Part model, mm, in its own coordinate system. A direction names the side the tool comes from. Give positions to 0.01 mm unless a question says otherwise; leave off trailing zeros. Order: outer loops, then holes, each group sorted by start corner. A loop starts at its lowest first (then second) coordinate and runs counter-clockwise, first axis right, second up. Notation, with made-up numbers: M -33.5,18 L -19.5,18 A25 cw -19.5,44 Z; hole C -17,-26 d2. An arc over 180 degrees is marked long. One line per question, with ' | ' between items.
```python
from build123d import *

# Parameters (mm, degrees)
SKETCH1_W           = 110
SKETCH1_H           = 45
BOSS_EXTRUDE1_DEPTH = 2
SKETCH3_W           = 110
SKETCH3_H           = 45
SKETCH3_W_2         = 106
SKETCH3_H_2         = 41
BOSS_EXTRUDE2_DEPTH = 30
SKETCH4_W           = 12
SKETCH4_H           = 41
BOSS_EXTRUDE3_DEPTH = 12
SKETCH5_W           = 6
SKETCH5_H           = 6
BOSS_EXTRUDE4_DEPTH = 18
SKETCH6_W           = 6
SKETCH6_H           = 6
BOSS_EXTRUDE5_DEPTH = 18
FILLET1_R           = 4
FILLET2_R           = 4
SKETCH7_R           = 1.3
CUT_EXTRUDE1_DEPTH  = 34
SKETCH8_R           = 2.9
CUT_EXTRUDE2_DEPTH  = 25
SKETCH9_W           = 10
SKETCH9_H           = 20
CUT_EXTRUDE3_DEPTH  = 10


with BuildPart() as part:
    # Sketch1 → Boss-Extrude1 (new body)
    with BuildSketch(Plane(origin=(0, 0, 0), x_dir=(1, 0, 0), z_dir=(0, 1, 0))):
        Rectangle(SKETCH1_W, SKETCH1_H)
    extrude(amount=BOSS_EXTRUDE1_DEPTH)

    # Sketch3 → Boss-Extrude2 (add)
    with BuildSketch(Plane(origin=(0, 2, 0), x_dir=(1, 0, 0), z_dir=(0, 1, 0))):
        Rectangle(SKETCH3_W, SKETCH3_H)
        Rectangle(SKETCH3_W_2, SKETCH3_H_2, mode=Mode.SUBTRACT)
    extrude(amount=BOSS_EXTRUDE2_DEPTH)

    # Sketch4 → Boss-Extrude3 (add)
    with BuildSketch(Plane(origin=(0, 2, 0), x_dir=(1, 0, 0), z_dir=(0, 1, 0))):
        with Locations((-47, 0)):
            Rectangle(SKETCH4_W, SKETCH4_H)
        with Locations((47, 0)):
            Rectangle(SKETCH4_W, SKETCH4_H)
    extrude(amount=BOSS_EXTRUDE3_DEPTH)

    # Sketch5 → Boss-Extrude4 (add)
    with BuildSketch(Plane(origin=(0, 14, 0), x_dir=(1, 0, 0), z_dir=(0, 1, 0))):
        with Locations((-50, 17.5)):
            Rectangle(SKETCH5_W, SKETCH5_H)
        with Locations((-50, -17.5)):
            Rectangle(SKETCH5_W, SKETCH5_H)
    extrude(amount=BOSS_EXTRUDE4_DEPTH)

    # Sketch6 → Boss-Extrude5 (add)
    with BuildSketch(Plane(origin=(0, 14, 0), x_dir=(1, 0, 0), z_dir=(0, 1, 0))):
        with Locations((50, 17.5)):
            Rectangle(SKETCH6_W, SKETCH6_H)
        with Locations((50, -17.5)):
            Rectangle(SKETCH6_W, SKETCH6_H)
    extrude(amount=BOSS_EXTRUDE5_DEPTH)

    # Fillet1
    fillet1_edges = [part.edges().sort_by_distance(p)[0] for p in [
        (55, 16, 22.5),
        (-55, 16, 22.5),
        (-55, 16, -22.5),
        (55, 16, -22.5),
    ]]
    fillet(fillet1_edges, radius=FILLET1_R)

    # Fillet2
    fillet2_edges = [part.edges().sort_by_distance(p)[0] for p in [
        (0, 0, -22.5),
        (55, 0, 0),
        (0, 0, 22.5),
        (-55, 0, 0),
        (-53.828427125, 0, -21.328427125),
        (-53.828427125, 0, 21.328427125),
        (53.828427125, 0, 21.328427125),
        (53.828427125, 0, -21.328427125),
    ]]
    fillet(fillet2_edges, radius=FILLET2_R)

    # Sketch7 → Cut-Extrude1 (cut)
    with BuildSketch(Plane(origin=(0, 32, 0), x_dir=(1, 0, 0), z_dir=(0, 1, 0))):
        with Locations(Location((-51, 18.5, 0), (0, 0, 270))):
            Circle(SKETCH7_R)
        with Locations(Location((51, 18.5, 0), (0, 0, 270))):
            Circle(SKETCH7_R)
        with Locations(Location((51, -18.5, 0), (0, 0, 270))):
            Circle(SKETCH7_R)
        with Locations(Location((-51, -18.5, 0), (0, 0, 270))):
            Circle(SKETCH7_R)
    extrude(amount=-CUT_EXTRUDE1_DEPTH, mode=Mode.SUBTRACT)

    # Sketch8 → Cut-Extrude2 (cut)
    with BuildSketch(Plane.XZ):
        with Locations(Location((-51, 18.5, 0), (0, 0, 270))):
            Circle(SKETCH8_R)
        with Locations(Location((-51, -18.5, 0), (0, 0, 270))):
            Circle(SKETCH8_R)
        with Locations(Location((51, -18.5, 0), (0, 0, 270))):
            Circle(SKETCH8_R)
        with Locations(Location((51, 18.5, 0), (0, 0, 270))):
            Circle(SKETCH8_R)
    extrude(amount=-CUT_EXTRUDE2_DEPTH, mode=Mode.SUBTRACT)

    # Sketch9 → Cut-Extrude3 (cut)
    with BuildSketch(Plane(origin=(0, 2, 0), x_dir=(1, 0, 0), z_dir=(0, 1, 0))):
        with Locations((36, 0)):
            Rectangle(SKETCH9_W, SKETCH9_H)
    extrude(amount=-CUT_EXTRUDE3_DEPTH, mode=Mode.SUBTRACT)


solid = part.part
```
1. Mould opens along Z. For faces 4 (the flat face through (-1, 18, -22.5)), 5 (the flat face through (55, 18, 0)), 6 (the flat face through (36, 1, -10)) say: released by +Z, released by -Z, zero draft, split by the parting line, or undercut.
Worked out:
face 4: released by -Z | face 5: zero draft | face 6: undercut
2. Slice it at C-C on x = -6. Give the cut face in (y, z).
Worked out:
outline: M 0,-18.5 A4 ccw 4,-22.5 L 32,-22.5 L 32,-20.5 L 2,-20.5 L 2,20.5 L 32,20.5 L 32,22.5 L 4,22.5 A4 ccw 0,18.5 Z
3. Probe L1, parallel to X at y = 16, z = -18.5; L2, parallel to X at y = 28, z = 18.5; L3, parallel to X at y = 5, z = -3.5. List the from-to ranges inside material, lowest first. Write a range as from..to.
Worked out:
L1: x = -55..-53.9, -48.1..-47, 47..48.1, 53.9..55 | L2: x = -55..-52.3, -49.7..-47, 47..49.7, 52.3..55 | L3: x = -55..-41, 41..55
4. Slice it at A-A on y = 26. Give the cut face in (x, z).
Worked out:
outline: M -55,-18.5 A4 ccw -51,-22.5 L 51,-22.5 A4 ccw 55,-18.5 L 55,18.5 A4 ccw 51,22.5 L -51,22.5 A4 ccw -55,18.5 Z; hole M -53,-14.5 L -47,-14.5 L -47,-20.5 L 47,-20.5 L 47,-14.5 L 53,-14.5 L 53,14.5 L 47,14.5 L 47,20.5 L -47,20.5 L -47,14.5 L -53,14.5 Z; hole C -51,-18.5 d2.6; hole C -51,18.5 d2.6; hole C 51,-18.5 d2.6; hole C 51,18.5 d2.6
5. Slice it at B-B on z = -8. Give the cut face in (x, y), then the cut area to 3 significant figures.
Worked out:
outline: M -55,4 A4 ccw -51,0 L 31,0 L 31,2 L -41,2 L -41,14 L -53,14 L -53,32 L -55,32 Z; M 41,0 L 51,0 A4 ccw 55,4 L 55,32 L 53,32 L 53,14 L 41,14 Z | area: 601 mm2
6. Slice it at D-D on y = 10. Give the cut face in (x, z), then the cut area to 3 significant figures.
Worked out:
outline: M -55,-18.5 A4 ccw -51,-22.5 L 51,-22.5 A4 ccw 55,-18.5 L 55,18.5 A4 ccw 51,22.5 L -51,22.5 A4 ccw -55,18.5 Z; hole C -51,-18.5 d5.8; hole C -51,18.5 d5.8; hole M -41,-20.5 L 41,-20.5 L 41,20.5 L -41,20.5 Z; hole C 51,-18.5 d5.8; hole C 51,18.5 d5.8 | area: 1,470 mm2
7. Drop flat-ended pins along their axis: pin 1 (12.5 mm diameter, centred on x = -18, z = 4, fed in from +Y); pin 2 (3 mm diameter, centred on x = -51.5, z = 19, fed in from -Y); pin 3 (0.6 mm diameter, centred on x = 38, y = 1, fed in from -Z). Give the stop position or say it passes through.
Worked out:
pin 1: stops at y = 2 | pin 2: stops at y = 25 | pin 3: stops at z = -21.45
8. Tool access for faces 1 (the cylindrical face through (53.797, 18.196, 21.359)), 2 (the flat face through (-50, 23, 14.5)), 3 (the flat face through (50, 25, 17)): list every direction of +Z, -Z, +X, -X, +Y, -Y with a clear straight run to the whole face (end or side of a thin tool).
Worked out:
face 1: +Z, +X, +Y, -Y | face 2: +Y | face 3: -Y
